Check sheet for the drawn part. Datum: minimum x, y, z corner. Units: mm. Round coordinates to 2 decimals unless told otherwise and drop trailing zeros. Write each loop counter-clockwise with the first axis right and the second up, starting at its lowest first coordinate (ties: lowest second). Pieces come first, ordered by that corner, then holes. Notation, with made-up numbers: (-8, 59) - (42, 59) arc R7 ccw to (42, 71) - close; hole circle Ø11 at (86, 33.25). An arc over 180 degrees is marked (long way). Answer as a JSON object with one key per item and string values. Group by question number.
Item 1: Thickness scan on line 1 (X direction, y = 16, z = 1); line 2 (Y direction, x = 65, z = 1.3); line 3 (X direction, y = 61.5, z = 0.8). Record the ranges inside material, lowest first.
Item 2: Sectioned sample at C-C on z = 1.95. Record the boundary of the cut face in (x, y) (3 decimals), plus the area to 3 significant figures.
Item 3: Sectioned sample at D-D on x = 93.98. Record the boundary of the cut face in (y, z) (3 decimals), plus the area to 3 significant figures.
Item 4: Sectioned sample at A-A on x = 38.1. Record the boundary of the cut face in (y, z) (3 decimals), plus the area to 3 significant figures.
Item 5: Gauge pin test, flat end, axial feed: P1, Ø4, axis at x = 63.5, y = 15.875, coming from the -Z side. Record the tip position at first contact, or that the pin passes through.
Item 6: Sectioned sample at B-B on y = 38.1. Record the boundary of the cut face in (x, z) (3 decimals).
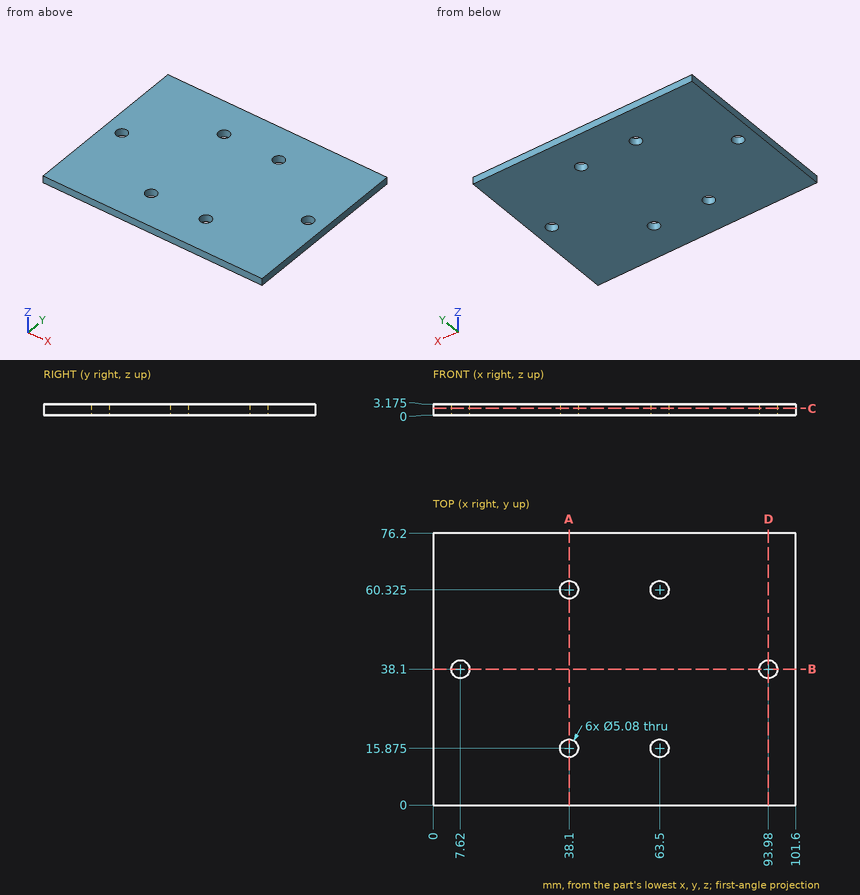
Completed:
{
 "1": {"line 1": "0 to 35.56, 40.64 to 60.96, 66.04 to 101.6", "line 2": "0 to 13.83, 17.92 to 58.28, 62.37 to 76.2", "line 3": "0 to 35.85, 40.35 to 61.25, 65.75 to 101.6"},
 "2": {"outline": "(0, 0) - (101.6, 0) - (101.6, 76.2) - (0, 76.2) - close; hole circle Ø5.08 at (7.62, 38.1); hole circle Ø5.08 at (38.1, 15.875); hole circle Ø5.08 at (38.1, 60.325); hole circle Ø5.08 at (63.5, 15.875); hole circle Ø5.08 at (63.5, 60.325); hole circle Ø5.08 at (93.98, 38.1)", "area": "7,620 mm²"},
 "3": {"outline": "(0, 0) - (35.56, 0) - (35.56, 3.175) - (0, 3.175) - close; (40.64, 0) - (76.2, 0) - (76.2, 3.175) - (40.64, 3.175) - close", "area": "226 mm²"},
 "4": {"outline": "(0, 0) - (13.335, 0) - (13.335, 3.175) - (0, 3.175) - close; (18.415, 0) - (57.785, 0) - (57.785, 3.175) - (18.415, 3.175) - close; (62.865, 0) - (76.2, 0) - (76.2, 3.175) - (62.865, 3.175) - close", "area": "210 mm²"},
 "5": {"P1": "through"},
 "6": {"outline": "(0, 0) - (5.08, 0) - (5.08, 3.175) - (0, 3.175) - close; (10.16, 0) - (91.44, 0) - (91.44, 3.175) - (10.16, 3.175) - close; (96.52, 0) - (101.6, 0) - (101.6, 3.175) - (96.52, 3.175) - close"}
}
